Read the model definition and answer for the solid it produces. Units are mm, in the model's axes. Give positions to 0.01 mm unless a question says otherwise; leave off trailing zeros. Loops run counter-clockwise (first coordinate to the right, second up) from the corner with the lowest first, then second, coordinate; pieces in that order, holes last. Notation, with made-up numbers: (42.25, 2) -> (72.25, 2) arc R30 ccw to (72.25, 33) -> close; hole circle Ø10 at (-8.75, -20). An arc over 180 degrees is marked (long way). Return JSON: item names as keys, results as strings. Group by question number.
from build123d import *

# Parameters (mm, degrees)
SKETCH1_W          = 523.3416
SKETCH1_H          = 101.6
SKETCH1_R          = 2.45745
BASE_FLANGE1_DEPTH = 3.175
HEM1_DEPTH         = 523.3416
HEM1_2_DEPTH       = 523.3416
FILLET1_R          = 3.175


# Read off the part's stored shape, not the designer's step: Hem1
# Sheet-metal steps are written as plain solids
with BuildPart() as part:
    # Sketch1 → Base-Flange1 (new body)
    with BuildSketch(Plane(origin=(0, 0, 0), x_dir=(0, 0, -1), z_dir=(1, 0, 0))):
        with Locations((-261.6708, 50.8)):
            Rectangle(SKETCH1_W, SKETCH1_H)
        with Locations((-510.15011, 76.2)):
            Circle(SKETCH1_R, mode=Mode.SUBTRACT)
        with Locations((-446.65011, 76.2)):
            Circle(SKETCH1_R, mode=Mode.SUBTRACT)
        with Locations((-446.65011, 25.4)):
            Circle(SKETCH1_R, mode=Mode.SUBTRACT)
        with Locations((-510.15011, 25.4)):
            Circle(SKETCH1_R, mode=Mode.SUBTRACT)
        with Locations(Location((-76.69149, 76.2, 0), (0, 0, 180))):
            Circle(SKETCH1_R, mode=Mode.SUBTRACT)
        with Locations(Location((-76.69149, 25.4, 0), (0, 0, 180))):
            Circle(SKETCH1_R, mode=Mode.SUBTRACT)
        with Locations(Location((-13.19149, 25.4, 0), (0, 0, 180))):
            Circle(SKETCH1_R, mode=Mode.SUBTRACT)
        with Locations(Location((-13.19149, 76.2, 0), (0, 0, 180))):
            Circle(SKETCH1_R, mode=Mode.SUBTRACT)
    extrude(amount=-BASE_FLANGE1_DEPTH)

    # Hem1 outline → Hem1 (cut)
    with BuildSketch(Plane.XY):
        with BuildLine():
            ThreePointArc((-3.175, 98.375), (-2.248029047, 100.637672645), (0, 101.59961238))
            Line((0, 101.59961238), (0, 101.6))
            Line((0, 101.6), (-3.175, 101.6))
            Line((-3.175, 101.6), (-3.175, 98.375))
        make_face()
        with BuildLine():
            ThreePointArc((0, 0.00038762), (-2.248029047, 0.962327355), (-3.175, 3.225))
            Line((-3.175, 3.225), (-3.175, 0))
            Line((-3.175, 0), (0, 0))
            Line((0, 0), (0, 0.00038762))
        make_face()
    extrude(amount=HEM1_DEPTH, mode=Mode.SUBTRACT)

    # Hem1 2 outline → Hem1 2 (add)
    with BuildSketch(Plane.XY):
        with BuildLine():
            Line((0.1, 88.9), (3.275, 88.9))
            Line((3.275, 88.9), (3.275, 98.375))
            ThreePointArc((3.275, 98.375), (2.312672645, 100.673029047), (0, 101.59961238))
            Line((0, 101.59961238), (0, 98.375))
            ThreePointArc((0, 98.375), (0.05, 98.425), (0.1, 98.375))
            Line((0.1, 98.375), (0.1, 88.9))
        make_face()
        with BuildLine():
            ThreePointArc((0.1, 3.225), (0.05, 3.175), (0, 3.225))
            Line((0, 3.225), (0, 0.00038762))
            ThreePointArc((0, 0.00038762), (2.312672645, 0.926970953), (3.275, 3.225))
            Line((3.275, 3.225), (3.275, 12.7))
            Line((3.275, 12.7), (0.1, 12.7))
            Line((0.1, 12.7), (0.1, 3.225))
        make_face()
    extrude(amount=HEM1_2_DEPTH)

    # Fillet1
    fillet1_edges = [part.edges().sort_by_distance(p)[0] for p in [
        (1.6875, 88.9, 523.3416),
        (1.6875, 88.9, 0),
        (1.6875, 12.7, 0),
        (1.6875, 12.7, 523.3416),
    ]]
    fillet(fillet1_edges, radius=FILLET1_R)


solid = part.part
1. Section A-A on z = 318 is taken. Determine the outline of the cut face in (x, y) (3 decimals).
2. Straight lines are drawn through the part: line 1 (Y direction, x = 0.75, z = 289); line 2 (Y direction, x = 0.5, z = 498); line 3 (X direction, y = 54, z = 430) (3 decimals). For each, find the intervals that lie inside material, in ascending order. Write a range as from..to.
3. Flat-ended cylindrical pins translate along their axes: pin 1 Ø1.6 at (x, z) = (1, 379) entering from +Y; pin 2 Ø8 at (y, z) = (26, 217.5) entering from +X; pin 3 Ø3.5 at (x, z) = (2.5, 198) entering from -Y. Find the tip coordinate at first contact, or state that the pin passes through.
4. Section C-C on y = 17.5 is taken. Determine the outline of the cut face in (x, z) (3 decimals).
5. Section B-B on x = 1.5 is taken. Determine the outline of the cut face in (y, z) (3 decimals), then the cut area to 3 significant figures.
Completed:
{
 "1": {"outline": "(-3.175, 3.225) arc R3.225 ccw to (3.275, 3.225) -> (3.275, 12.7) -> (0.1, 12.7) -> (0.1, 3.225) arc R0.05 cw to (0, 3.225) -> (0, 98.375) arc R0.05 cw to (0.1, 98.375) -> (0.1, 88.9) -> (3.275, 88.9) -> (3.275, 98.375) arc R3.225 ccw to (-3.175, 98.375) -> close"},
 "2": {"line 1": "y = 0.08..12.7, 88.9..101.52", "line 2": "y = 0.03..12.7, 88.9..101.57", "line 3": "x = -3.175..0"},
 "3": {"pin 1": "stops at y = 101.6", "pin 2": "stops at x = 0", "pin 3": "stops at y = 0.08"},
 "4": {"outline": "(-3.175, 0) -> (0, 0) -> (0, 523.342) -> (-3.175, 523.342) -> close"},
 "5": {"outline": "(0.344, 0) -> (9.525, 0) arc R3.175 ccw to (12.7, 3.175) -> (12.7, 520.167) arc R3.175 ccw to (9.525, 523.342) -> (0.344, 523.342) -> close; (88.9, 3.175) arc R3.175 ccw to (92.075, 0) -> (101.256, 0) -> (101.256, 523.342) -> (92.075, 523.342) arc R3.175 ccw to (88.9, 520.167) -> close", "area": "12,900 mm²"}
}
